```python
from build123d import *

# Parameters (mm, degrees)
SKETCH1_W             = 33.02
SKETCH1_H             = 4.826
BOSS_EXTRUDE1_DEPTH   = 3.302
SKETCH2_W             = 6.096
SKETCH2_H             = 3.302
BOSS_EXTRUDE2_DEPTH   = 12.446
F_6_32_TAPPED_HOLE1_D = 2.7051
F_6_32_TAPPED_HOLE2_D = 2.7051


with BuildPart() as part:
    # Sketch1 → Boss-Extrude1 (new body)
    with BuildSketch(Plane(origin=(0, 0, 0), x_dir=(0, 0, -1), z_dir=(1, 0, 0))):
        with Locations((16.51, 2.413)):
            Rectangle(SKETCH1_W, SKETCH1_H)
    extrude(amount=BOSS_EXTRUDE1_DEPTH)

    # Sketch2 → Boss-Extrude2 (add)
    with BuildSketch(Plane.ZY):
        with Locations((-29.972, 6.477)):
            Rectangle(SKETCH2_W, SKETCH2_H)
        with Locations((-3.048, 6.477)):
            Rectangle(SKETCH2_W, SKETCH2_H)
    extrude(amount=-BOSS_EXTRUDE2_DEPTH)

    # #6-32 Tapped Hole1 (through all)
    with Locations(Plane(origin=(3.302, 0, 0), x_dir=(0, 0, -1), z_dir=(1, 0, 0))):
        with Locations((3.0353, 3.302), (29.9847, 3.302)):
            Hole(F_6_32_TAPPED_HOLE1_D / 2)

    # #6-32 Tapped Hole2 (through all)
    with Locations(Plane(origin=(0, 8.128, 0), x_dir=(1, 0, 0), z_dir=(0, 1, 0))):
        with Locations((9.398, 3.0353), (9.398, 29.9847)):
            Hole(F_6_32_TAPPED_HOLE2_D / 2)


solid = part.part
```
Read the model definition and answer for the solid it produces. Units are mm, in the model's axes. A direction names the side the tool comes from. Give positions to 0.01 mm unless a question says otherwise; leave off trailing zeros. Write each loop counter-clockwise with the first axis right and the second up, starting at its lowest first coordinate (ties: lowest second). Pieces come first, ordered by that corner, then holes. Notation, with made-up numbers: (33.5, 48) -> (41.5, 48) arc R20 cw to (41.5, 84) -> close; hole circle Ø10 at (68, 35). An arc over 180 degrees is marked (long way). Answer in a Markdown table with one row per item.
1) Each of these flat-tipped pins is pushed along its axis until it touches: pin 1 Ø1.5 at (y, z) = (4, -10) entering from +X; pin 2 Ø3 at (x, z) = (9.4, -3.04) entering from -Y; pin 3 Ø2.5 at (y, z) = (3.3, -29.98) entering from -X; pin 4 Ø1.7 at (x, z) = (2, -17.5) entering from +Y. Where does it stop, or does it pass through?
Results list:
| item | result |
|---|---|
| pin 1 | x = 3.3 |
| pin 2 | y = 4.83 |
| pin 3 | through |
| pin 4 | y = 4.83 |
2) Determine the mould class of faces 1 (the flat face through (0, 3, -17)), 2 (the flat face through (12.446, 7, -3)), 3 (the cylindrical face through (8.774, 6.454, -28.785)), 4 (the cylindrical face through (8.774, 6.454, -1.835)) for opening direction X: released by +X, released by -X, zero draft, split by the parting line, or undercut.
Results list:
| item | result |
|---|---|
| face 1 | released by -X |
| face 2 | released by +X |
| face 3 | undercut |
| face 4 | undercut |
3) Section B-B on y = 5.5 is taken. Give the vertices of the cut face in (x, z).
Results list:
| item | result |
|---|---|
| outline | (0, -33.02) -> (12.45, -33.02) -> (12.45, -26.92) -> (0, -26.92) -> close; (0, -6.1) -> (12.45, -6.1) -> (12.45, 0) -> (0, 0) -> close; hole circle Ø2.71 at (9.4, -29.98); hole circle Ø2.71 at (9.4, -3.04) |
4) Section C-C on x = 4.5 is taken. Give the vertices of the cut face in (y, z), plus the area to 3 significant figures.
Results list:
| item | result |
|---|---|
| outline | (4.83, -33.02) -> (8.13, -33.02) -> (8.13, -26.92) -> (4.83, -26.92) -> close; (4.83, -6.1) -> (8.13, -6.1) -> (8.13, 0) -> (4.83, 0) -> close |
| area | 40.3 mm^2 |
5) Section A-A on x = 3 is taken. Give the vertices of the cut face in (y, z).
Results list:
| item | result |
|---|---|
| outline | (0, -33.02) -> (8.13, -33.02) -> (8.13, -26.92) -> (4.83, -26.92) -> (4.83, -6.1) -> (8.13, -6.1) -> (8.13, 0) -> (0, 0) -> close; hole circle Ø2.71 at (3.3, -29.98); hole circle Ø2.71 at (3.3, -3.04) |
6) A tool of negligible diameter and unlimited length cuts with its end or side. For faces 5 (the flat face through (7.8, 4.826, -30)), 6 (the flat face through (6, 8.128, -3)), 7 (the flat face through (2, 4.826, -16)), from which of +Z, -Z, +X, -X, +Y, -Y can it reach the whole face along a straight path? Write none if from no direction.
Results list:
| item | result |
|---|---|
| face 5 | +Z, -Z, +X, -Y |
| face 6 | +Z, -Z, +X, -X, +Y |
| face 7 | +X, -X, +Y |
7) Section D-D on y = 2.5 is taken. Give the vertices of the cut face in (x, z).
Results list:
| item | result |
|---|---|
| outline | (0, -33.02) -> (3.3, -33.02) -> (3.3, -31.07) -> (0, -31.07) -> close; (0, -28.9) -> (3.3, -28.9) -> (3.3, -4.12) -> (0, -4.12) -> close; (0, -1.95) -> (3.3, -1.95) -> (3.3, 0) -> (0, 0) -> close |
8) Straight lines are drawn through the part: line 1 (Z direction, x = 4.75, y = 5.75); line 2 (X direction, y = 2, z = -24.5); line 3 (Y direction, x = 2, z = -9.5). For each, find the intervals that lie inside material, in ascending order. Write a range as [from, to].
Results list:
| item | result |
|---|---|
| line 1 | [-33.02, -26.92], [-6.1, 0] |
| line 2 | [0, 3.3] |
| line 3 | [0, 4.83] |
